from build123d import *

# Parameters (mm, degrees)
F0_W     = 203.2
F0_H     = 127
F1_DEPTH = 12.7
F2_W     = 203.2
F2_H     = 12.7
F3_DEPTH = 25.4
F5_DEPTH = 127
F6_W     = 203.2
F6_H     = 12.7
F7_DEPTH = 25.4
F9_DEPTH = 50.8


with BuildPart() as f1:
    # F0 (on Top) → F1 (new body, symmetric)
    with BuildSketch(Plane.XY):
        Rectangle(F0_W, F0_H)
    extrude(amount=F1_DEPTH, both=True)

    # F2 (on face) → F3 (join)
    with BuildSketch(Plane.XY.offset(12.7)):
        with Locations((0, 57.15)):
            Rectangle(F2_W, F2_H)
        with Locations((0, -57.15)):
            Rectangle(F2_W, F2_H)
    extrude(amount=F3_DEPTH)

    # F4 (on face) → F5 (cut)
    with BuildSketch(Plane.XZ.offset(63.5)):
        with BuildLine():
            Line((-88.9, 19.05), (88.9, 19.05))
            ThreePointArc((88.9, 19.05), (95.25, 25.4), (88.9, 31.75))
            Line((88.9, 31.75), (-88.9, 31.75))
            ThreePointArc((-88.9, 31.75), (-95.25, 25.4), (-88.9, 19.05))
        make_face()
    extrude(amount=-F5_DEPTH, mode=Mode.SUBTRACT)

    # F6 (on face) → F7 (join)
    with BuildSketch(Plane.XY.offset(12.7)):
        with Locations((0, 19.05)):
            Rectangle(F6_W, F6_H)
        with Locations((0, -19.05)):
            Rectangle(F6_W, F6_H)
    extrude(amount=F7_DEPTH)

    # F8 (on face) → F9 (cut)
    with BuildSketch(Plane(origin=(0, 25.4, 0), x_dir=(-1, 0, 0), z_dir=(0, 1, 0))):
        with BuildLine():
            Line((88.9, 31.75), (-88.9, 31.75))
            ThreePointArc((-88.9, 31.75), (-95.25, 25.4), (-88.9, 19.05))
            Line((-88.9, 19.05), (88.9, 19.05))
            ThreePointArc((88.9, 19.05), (95.25, 25.4), (88.9, 31.75))
        make_face()
    extrude(amount=-F9_DEPTH, mode=Mode.SUBTRACT)


solid = f1.part
Geometry: final body of the model. Coordinates: model frame, mm. A direction names the side the tool comes from. Give positions to 0.01 mm unless a question says otherwise; leave off trailing zeros. Order: outer loops, then holes, each group sorted by start corner. A loop starts at its lowest first (then second) coordinate and runs counter-clockwise, first axis right, second up. Notation, with made-up numbers: (66.25, 76.25) -> (90.25, 76.25) arc R19 ccw to (90.25, 90.25) -> close; hole circle Ø2 at (74.25, 81). An arc over 180 degrees is marked (long way). Write each question's results on one line, items separated by ' | '.
1) Line query: line 1 along Y through (x, z) = (83, 17.5); line 2 along Z through (x, y) = (88.5, 43); line 3 along Z through (x, y) = (-5, 51.5). Output: solid intervals per line, ascending.
Geometry says:
line 1: y = -63.5 to -50.8, -25.4 to -12.7, 12.7 to 25.4, 50.8 to 63.5 | line 2: z = -12.7 to 12.7 | line 3: z = -12.7 to 19.05, 31.75 to 38.1
2) Cut plane A-A (z = 25.4). Give the number of separate pieces and of enclosed holes in the cut face, and give its area (3 significant figures).
Geometry says:
separate pieces: 8 | enclosed holes: 0 | area: 645 mm²
3) First-contact query: pin 1 Ø12.5 at (x, y) = (-39, -35) entering from +Z. Flat tip, straight axial feed; report the tip coordinate or a pass-through.
Geometry says:
pin 1: stops at z = 12.7
4) Cut plane C-C (y = -16). Output: boundary loops of the cut face in (x, z), and give its area (3 significant figures).
Geometry says:
outline: (-101.6, -12.7) -> (101.6, -12.7) -> (101.6, 38.1) -> (-101.6, 38.1) -> close; hole (-88.9, 19.05) -> (88.9, 19.05) arc R6.35 ccw to (88.9, 31.75) -> (-88.9, 31.75) arc R6.35 ccw to start | area: 7,940 mm²
5) Draft query along Y for faces 4 (the face through (-1, 38, 12.7)), 5 (the face through (95.25, 57.06, 25.26)), 6 (the face through (-1, 63.5, 7)). Return one class per face: released by +Y, released by -Y, zero draft, split by the parting line, or undercut.
Geometry says:
face 4: undercut | face 5: zero draft | face 6: released by +Y
6) Set-up query: faces 1 (the face through (-95.25, 57.06, 25.54)), 2 (the face through (-1, 50.8, 17)), 3 (the face through (101.6, -1, 7)). Return all of +Z, -Z, +X, -X, +Y, -Y with unobstructed straight access to the full face (end or side cutting, diameter ignored); none if empty.
Geometry says:
face 1: +Y, -Y | face 2: +Z, +X, -X | face 3: +Z, -Z, +X, +Y, -Y
